from build123d import *

# Parameters (mm, degrees)
BOSS_EXTRUDE1_DEPTH     = 1.5
SKETCH2_W               = 6.5
SKETCH2_H               = 41.6
BOSS_EXTRUDE2_DEPTH     = 2
SKETCH3_W               = 6.5
SKETCH3_H               = 22.029549655
BOSS_EXTRUDE3_DEPTH     = 2
CUT_EXTRUDE1_DEPTH      = 66.428669726
CUT_EXTRUDE1_DEPTH_BACK = 66.428669726
FILLET1_R               = 2
FILLET2_R               = 1.5


# Some blends are built 0.0001 mm under size
with BuildPart() as part:
    # Sketch1 → Boss-Extrude1 (new, symmetric)
    with BuildSketch(Plane(origin=(0, 0, 0), x_dir=(0, 0, -1), z_dir=(1, 0, 0))):
        Polygon((-43.305040632, 32.259635184), (-38.1, 0), (0, 0), (-31.3944757, 46.45409373), align=None)
    extrude(amount=BOSS_EXTRUDE1_DEPTH, both=True)

    # Sketch2 → Boss-Extrude2 (add)
    with BuildSketch(Plane.XZ):
        with Locations((0, 19.05)):
            Rectangle(SKETCH2_W, SKETCH2_H)
    extrude(amount=-BOSS_EXTRUDE2_DEPTH)

    # Sketch3 → Boss-Extrude3 (add)
    with BuildSketch(Plane(origin=(0, 34.65247404, 41.29721043), x_dir=(1, 0, 0), z_dir=(0, 0.6427876096865434, 0.7660444431189747))):
        with Locations((0, 6.141145543)):
            Rectangle(SKETCH3_W, SKETCH3_H)
    extrude(amount=-BOSS_EXTRUDE3_DEPTH)

    # Sketch4 → Cut-Extrude1 (cut, two sides: drawn at the far end of the back side and taken through both)
    with BuildSketch(Plane(origin=(1.5, 0, 0), x_dir=(0, 0, -1), z_dir=(1, 0, 0)).offset(-CUT_EXTRUDE1_DEPTH_BACK)):
        Polygon((-36.523365649, 27.895930093), (-33.313189095, 8), (-12.648239091, 8), (-30.746767143, 34.780212116), align=None)
    extrude(amount=CUT_EXTRUDE1_DEPTH + CUT_EXTRUDE1_DEPTH_BACK, mode=Mode.SUBTRACT)

    # Fillet1
    # the kernel refuses this fillet: 2 mm, written as the material it adds along each edge
    with BuildSketch(Plane(origin=(1.5, 34.780212116, 30.746767143), x_dir=(0, -0.8285345686504685, -0.5599379149076996), z_dir=(-1, 0, 0))) as fillet1_piece_1:
        with BuildLine():
            CenterArc((FILLET1_R * 1.32580458231, FILLET1_R), FILLET1_R, 164.051504254, 105.948495746)
            Line((FILLET1_R * 0.364295499179, FILLET1_R * 1.27477314835), (0, 0))
            Line((0, 0), (FILLET1_R * 1.32580458231, 0))
        make_face()
    extrude(amount=3)
    with BuildSketch(Plane(origin=(-1.5, 8, 12.648239091), x_dir=(0, 0, 1), z_dir=(1, 0, 0))) as fillet1_piece_2:
        with BuildLine():
            CenterArc((FILLET1_R * 1.88276744741, -FILLET1_R), FILLET1_R, 90, 124.051504254)
            Line((FILLET1_R * 1.05423287876, -FILLET1_R * 1.55993791491), (0, 0))
            Line((0, 0), (FILLET1_R * 1.88276744741, 0))
        make_face()
    extrude(amount=3)
    with BuildSketch(Plane(origin=(1.5, 27.895930093, 36.523365649), x_dir=(0, 0.7660444431189765, -0.6427876096865413), z_dir=(-1, 0, 0))) as fillet1_piece_3:
        with BuildLine():
            CenterArc((FILLET1_R * 0.457472572927, FILLET1_R), FILLET1_R, 220.834409573, 49.165590427)
            Line((-FILLET1_R * 0.299129927729, FILLET1_R * 0.346124892658), (0, 0))
            Line((0, 0), (FILLET1_R * 0.457472572927, 0))
        make_face()
    extrude(amount=3)
    with BuildSketch(Plane(origin=(-1.5, 8, 33.313189095), x_dir=(0, 0, -1), z_dir=(1, 0, 0))) as fillet1_piece_4:
        with BuildLine():
            CenterArc((FILLET1_R * 0.851584618699, FILLET1_R), FILLET1_R, 189.165590427, 80.834409573)
            Line((-FILLET1_R * 0.135647486653, FILLET1_R * 0.840711676004), (0, 0))
            Line((0, 0), (FILLET1_R * 0.851584618699, 0))
        make_face()
    extrude(amount=3)
    # the kernel refuses this fillet: 2 mm, written as the material it takes off along each edge
    with BuildSketch(Plane(origin=(-1.5, 34.586150343, 43.680420138), x_dir=(0, 0.1592883239956265, -0.9872321053524669), z_dir=(0, -0.987232105352467, -0.15928832399562654))) as fillet1_2_piece_1_section:
        with BuildLine():
            CenterArc((FILLET1_R, FILLET1_R), FILLET1_R, 180, 90)
            Line((0, FILLET1_R), (0, 0))
            Line((0, 0), (FILLET1_R, 0))
        make_face()
    fillet1_2_piece_1 = extrude(amount=38.007587746, mode=Mode.PRIVATE)
    fillet1_2_piece_1 = split(fillet1_2_piece_1, bisect_by=Plane(origin=(-1.056244864, 22.976919754, 48.483349146), z_dir=(0, -0.6427876096865434, -0.7660444431189747)), keep=Keep.TOP, mode=Mode.PRIVATE)
    fillet1_2_piece_1 = split(fillet1_2_piece_1, bisect_by=Plane(origin=(-1.056244864, 2, 40.232595457), z_dir=(0, 1, 0)), keep=Keep.TOP, mode=Mode.PRIVATE)
    add(fillet1_2_piece_1, mode=Mode.SUBTRACT)
    with BuildSketch(Plane(origin=(-1.5, -2.142672843, -1.448055168), x_dir=(1, 0, 0), z_dir=(0, 0.8285345686504687, 0.5599379149076993))) as fillet1_2_piece_2_section:
        with BuildLine():
            CenterArc((FILLET1_R, -FILLET1_R), FILLET1_R, 90, 90)
            Line((0, -FILLET1_R), (0, 0))
            Line((0, 0), (FILLET1_R, 0))
        make_face()
    fillet1_2_piece_2 = extrude(amount=61.573815732, mode=Mode.PRIVATE)
    fillet1_2_piece_2 = split(fillet1_2_piece_2, bisect_by=Plane(origin=(-1.05170861, 38.993973381, 35.043445356), z_dir=(0, -0.6427876096865434, -0.7660444431189747)), keep=Keep.TOP, mode=Mode.PRIVATE)
    fillet1_2_piece_2 = split(fillet1_2_piece_2, bisect_by=Plane(origin=(-1.05170861, 2, 16.20714214), z_dir=(0, 1, 0)), keep=Keep.TOP, mode=Mode.PRIVATE)
    add(fillet1_2_piece_2, mode=Mode.SUBTRACT)
    with BuildSketch(Plane(origin=(1.5, -2.142672843, -1.448055168), x_dir=(0, -0.5599379149076993, 0.8285345686504687), z_dir=(0, 0.8285345686504687, 0.5599379149076993))) as fillet1_2_piece_3_section:
        with BuildLine():
            CenterArc((FILLET1_R, -FILLET1_R), FILLET1_R, 90, 90)
            Line((0, -FILLET1_R), (0, 0))
            Line((0, 0), (FILLET1_R, 0))
        make_face()
    fillet1_2_piece_3 = extrude(amount=61.573815732, mode=Mode.PRIVATE)
    fillet1_2_piece_3 = split(fillet1_2_piece_3, bisect_by=Plane(origin=(1.05170861, 38.993973381, 35.043445356), z_dir=(0, -0.6427876096865434, -0.7660444431189747)), keep=Keep.TOP, mode=Mode.PRIVATE)
    fillet1_2_piece_3 = split(fillet1_2_piece_3, bisect_by=Plane(origin=(1.05170861, 2, 16.20714214), z_dir=(0, 1, 0)), keep=Keep.TOP, mode=Mode.PRIVATE)
    add(fillet1_2_piece_3, mode=Mode.SUBTRACT)
    with BuildSketch(Plane(origin=(1.5, 34.586150343, 43.680420138), x_dir=(0, 0.1592883239956265, -0.9872321053524669), z_dir=(0, -0.987232105352467, -0.15928832399562654))) as fillet1_2_piece_4_section:
        with BuildLine():
            CenterArc((FILLET1_R, -FILLET1_R), FILLET1_R, 90, 90)
            Line((0, -FILLET1_R), (0, 0))
            Line((0, 0), (FILLET1_R, 0))
        make_face()
    fillet1_2_piece_4 = extrude(amount=38.007587746, mode=Mode.PRIVATE)
    fillet1_2_piece_4 = split(fillet1_2_piece_4, bisect_by=Plane(origin=(1.056244864, 22.976919754, 48.483349146), z_dir=(0, -0.6427876096865434, -0.7660444431189747)), keep=Keep.TOP, mode=Mode.PRIVATE)
    fillet1_2_piece_4 = split(fillet1_2_piece_4, bisect_by=Plane(origin=(1.056244864, 2, 40.232595457), z_dir=(0, 1, 0)), keep=Keep.TOP, mode=Mode.PRIVATE)
    add(fillet1_2_piece_4, mode=Mode.SUBTRACT)
    with BuildSketch(Plane(origin=(-3.25, 51.008609554, 34.099819599), x_dir=(0, -0.7660444431189747, 0.6427876096865432), z_dir=(0, -0.6427876096865434, -0.7660444431189747)), Plane(origin=(-3.25, -5, 39.85), x_dir=(0, 0, -1), z_dir=(0, 1, 0)), Plane(origin=(3.25, -5, 39.85), x_dir=(-1, 0, 0), z_dir=(0, 1, 0))) as fillet1_2_piece_5:
        with BuildLine():
            CenterArc((FILLET1_R, -FILLET1_R), FILLET1_R, 90, 90)
            Line((0, -FILLET1_R), (0, 0))
            Line((0, 0), (FILLET1_R, 0))
        make_face()
    extrude(amount=12, mode=Mode.SUBTRACT)
    with BuildSketch(Plane(origin=(-3.25, 34.132995457, 48.260141164), x_dir=(0, 0.7660444431189747, -0.6427876096865434), z_dir=(0, -0.6427876096865434, -0.7660444431189747)), Plane(origin=(3.25, 34.132995457, 48.260141164), x_dir=(-1, 0, 0), z_dir=(0, -0.6427876096865434, -0.7660444431189747))) as fillet1_2_piece_6:
        with BuildLine():
            CenterArc((FILLET1_R, FILLET1_R), FILLET1_R, 180, 90)
            Line((0, FILLET1_R), (0, 0))
            Line((0, 0), (FILLET1_R, 0))
        make_face()
    extrude(amount=7, mode=Mode.SUBTRACT)
    with BuildSketch(Plane(origin=(3.25, 51.008609554, 34.099819599), x_dir=(0, -0.7660444431189747, 0.6427876096865432), z_dir=(0, -0.6427876096865434, -0.7660444431189747)), Plane(origin=(-3.25, -5, -1.75), x_dir=(0, 0, 1), z_dir=(0, 1, 0)), Plane(origin=(3.25, -5, -1.75), x_dir=(-1, 0, 0), z_dir=(0, 1, 0))) as fillet1_2_piece_7:
        with BuildLine():
            CenterArc((FILLET1_R, FILLET1_R), FILLET1_R, 180, 90)
            Line((0, FILLET1_R), (0, 0))
            Line((0, 0), (FILLET1_R, 0))
        make_face()
    extrude(amount=12, mode=Mode.SUBTRACT)

    # Fillet2
    fillet2_edges = [part.edges().sort_by_distance(p)[0] for p in [
        (1.5, 9.061850667, 14.647456961),
        (1.5, 21.851569045, 22.009367742),
        (1.5, 33.460692344, 30.815325558),
        (1.5, 30.672890194, 34.193219453),
        (1.5, 27.842934726, 36.331192599),
        (1.5, 18.337045111, 34.981054819),
        (1.5, 8.477312689, 32.906716951),
        (-1.5, 9.061850667, 14.647456961),
        (-1.5, 21.851569045, 22.009367742),
        (-1.5, 33.460692344, 30.815325558),
        (-1.5, 30.672890194, 34.193219453),
        (-1.5, 27.842934726, 36.331192599),
        (-1.5, 18.337045111, 34.981054819),
        (-1.5, 8.477312689, 32.906716951),
        (1.5, 8, 24.011896921),
        (-1.5, 8, 24.011896921),
    ]]
    fillet(fillet2_edges, radius=FILLET2_R - 0.0001)  # a hair under: the kernel refuses the full size


solid = part.part
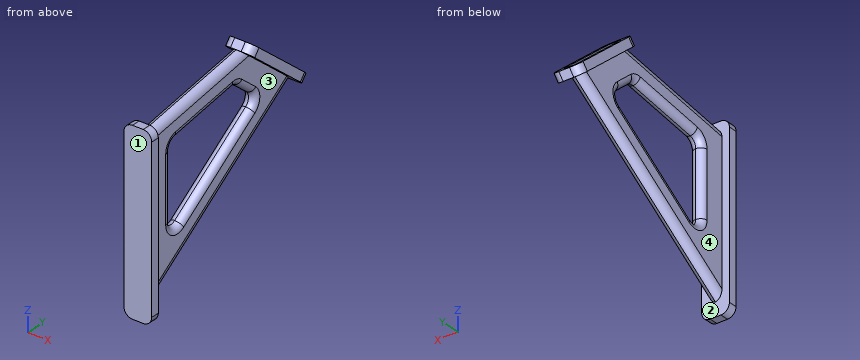
Geometry: final body of the model. Coordinates: model frame, mm. Face numbers are marked on the shaded views. A direction names the side the tool comes from. Give positions to 0.01 mm unless a question says otherwise; leave off trailing zeros. Write each loop counter-clockwise with the first axis right and the second up, starting at its lowest first coordinate (ties: lowest second). Pieces come first, ordered by that corner, then holes. Notation, with made-up numbers: (79, -36) -> (91, -36) arc R25 ccw to (91, -3) -> close; hole circle Ø3 at (-36, -26.75). An arc over 180 degrees is marked (long way). Answer in a Markdown table with one row per item.
(1) Set-up query: the marked faces 3 and 4. Return all of +Z, -Z, +X, -X, +Y, -Y with unobstructed straight access to the full face (end or side cutting, diameter ignored); none if empty.
Answers below:
| item | result |
|---|---|
| face 3 | -Z, +X |
| face 4 | -Z, -X |
(2) Ray query, line 1 along X through (y, z) = (3, 35); line 2 along Y through (x, z) = (-1.75, 15); line 3 along Y through (x, z) = (-0.25, 33). Return the intervals inside material, ascending. Write a range as [from, to].
Answers below:
| item | result |
|---|---|
| line 1 | [-1.5, 1.5] |
| line 2 | [0, 2] |
| line 3 | [0, 8.53], [32.13, 44.54] |
(3) Section query A-A on x = 2.5. Return loops of the section in (y, z).
Answers below:
| item | result |
|---|---|
| outline | (0, -1.31) -> (2, -1.31) -> (2, 39.41) -> (0, 39.41) -> close; (29.97, 42.62) -> (46.17, 29.02) -> (47.46, 30.55) -> (31.26, 44.15) -> close |
(4) Pin query (flat end, axial travel): pin 1 (3 mm diameter, centred on x = -1, z = 27, fed in from +Y); pin 2 (2 mm diameter, centred on x = -1, z = 35, fed in from +Y); pin 3 (1 mm diameter, centred on x = 1.5, y = 35.5, fed in from +Z); pin 4 (1 mm diameter, centred on x = 0.5, z = 30.5, fed in from -Y). Return the tip coordinate at first contact, or that it passes through.
Answers below:
| item | result |
|---|---|
| pin 1 | y = 41.62 |
| pin 2 | y = 43.35 |
| pin 3 | z = 41.01 |
| pin 4 | y = 0 |
(5) Draft query along Y for the marked faces 1 and 2. Return one class per face: +Y half, -Y half, draft (parallel to the pull), parting line (faces both ways), or undercut.
Answers below:
| item | result |
|---|---|
| face 1 | -Y half |
| face 2 | undercut |
